Verification items for the finished model (mm, model axes). Face numbers are marked on the shaded views. A direction names the side the tool comes from. Round coordinates to 2 decimals unless told otherwise and drop trailing zeros. Write each loop counter-clockwise with the first axis right and the second up, starting at its lowest first coordinate (ties: lowest second). Pieces come first, ordered by that corner, then holes. Notation, with made-up numbers: M -31,82 L -5,82 A23 cw -5,95 Z; hole C 50.25,39.5 d1. An arc over 180 degrees is marked long. One line per question, with ' | ' between items.
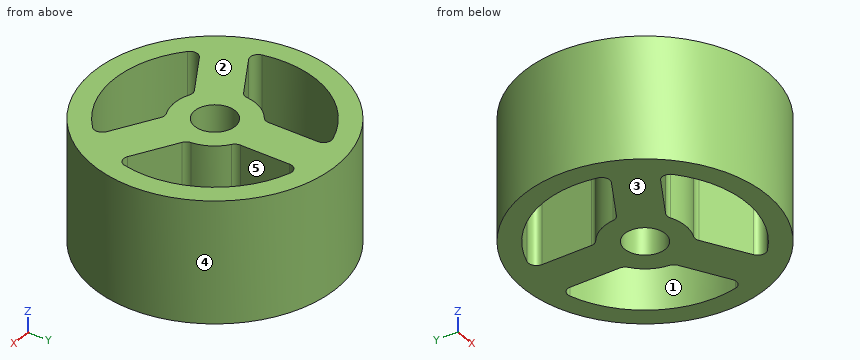
from build123d import *

# Parameters (mm, degrees)
SKETCH1_R           = 30
SKETCH1_R_2         = 25
SKETCH1_R_3         = 10
SKETCH1_R_4         = 5
BOSS_EXTRUDE1_DEPTH = 30


with BuildPart() as part:
    # Sketch1 → Boss-Extrude1 (new body)
    # profile 1 of 5: a face of its own
    with BuildSketch(Plane.XY):
        Circle(SKETCH1_R)
        Circle(SKETCH1_R_2, mode=Mode.SUBTRACT)
    # profile 2 of 5: a face of its own
    with BuildSketch(Plane.XY):
        with BuildLine():
            ThreePointArc((-7.608695652, 23.814024239), (-5.820464351, 23.524048006), (-5, 21.9089023))
            Line((-5, 21.9089023), (-5, 9.746794345))
            ThreePointArc((-5, 9.746794345), (-5.220486958, 8.833923416), (-5.833333333, 8.122328621))
            ThreePointArc((-5.833333333, 8.122328621), (0, 10), (5.833333333, 8.122328621))
            ThreePointArc((5.833333333, 8.122328621), (5.220486958, 8.833923416), (5, 9.746794345))
            Line((5, 9.746794345), (5, 21.9089023))
            ThreePointArc((5, 21.9089023), (5.820464351, 23.524048006), (7.608695652, 23.814024239))
            ThreePointArc((7.608695652, 23.814024239), (0, 25), (-7.608695652, 23.814024239))
        make_face()
    # profile 3 of 5: a face of its own
    with BuildSketch(Plane.XY):
        with BuildLine():
            ThreePointArc((-21.473665961, -6.624324131), (-23.282655349, -6.721354014), (-24.427897784, -5.317688395))
            ThreePointArc((-24.427897784, -5.317688395), (-21.650635095, -12.5), (-16.819202132, -18.496335844))
            ThreePointArc((-16.819202132, -18.496335844), (-17.462190998, -16.802693993), (-16.473665961, -15.284578169))
            Line((-16.473665961, -15.284578169), (-5.940971508, -9.203524191))
            ThreePointArc((-5.940971508, -9.203524191), (-5.040158614, -8.938036034), (-4.117476257, -9.112979166))
            ThreePointArc((-4.117476257, -9.112979166), (-8.660254038, -5), (-9.95080959, 0.990650545))
            ThreePointArc((-9.95080959, 0.990650545), (-10.260645572, 0.104112618), (-10.940971508, -0.543270153))
            Line((-10.940971508, -0.543270153), (-21.473665961, -6.624324131))
        make_face()
    # profile 4 of 5: a face of its own
    with BuildSketch(Plane.XY):
        with BuildLine():
            ThreePointArc((10.940971508, -0.543270153), (10.260645572, 0.104112618), (9.95080959, 0.990650545))
            ThreePointArc((9.95080959, 0.990650545), (9.987694827, 0.49593553), (10, 0))
            ThreePointArc((10, 0), (8.40162968, -5.423340181), (4.117476257, -9.112979166))
            ThreePointArc((4.117476257, -9.112979166), (5.040158614, -8.938036034), (5.940971508, -9.203524191))
            Line((5.940971508, -9.203524191), (16.473665961, -15.284578169))
            ThreePointArc((16.473665961, -15.284578169), (17.462190998, -16.802693993), (16.819202132, -18.496335844))
            ThreePointArc((16.819202132, -18.496335844), (21.650635095, -12.5), (24.427897784, -5.317688395))
            ThreePointArc((24.427897784, -5.317688395), (23.282655349, -6.721354014), (21.473665961, -6.624324131))
            Line((21.473665961, -6.624324131), (10.940971508, -0.543270153))
        make_face()
    # profile 5 of 5: a face of its own
    with BuildSketch(Plane.XY):
        Circle(SKETCH1_R_3)
        Circle(SKETCH1_R_4, mode=Mode.SUBTRACT)
    extrude(amount=BOSS_EXTRUDE1_DEPTH)


solid = part.part
1. Go/stop test with flat-tipped pins: P1, Ø10, axis at y = -17, z = 16.5, coming from the -X side; P2, Ø1, axis at y = -11, z = 25.5, coming from the -X side; P3, Ø1, axis at x = -17.5, y = -4, coming from the +Z side; P4, Ø6, axis at y = 16, z = 22, coming from the -X side. Record where each tip stops, or that it passes through.
Results:
P1: stops at x = -27.5 | P2: stops at x = -28.1 | P3: stops at z = 30 | P4: stops at x = -27.04
2. Tool access check on the marked faces 1 and 2. Record the directions out of +Z, -Z, +X, -X, +Y, -Y that give a thin tool (end or side, any length) a straight path to the whole face; none if there is none.
Results:
face 1: +Z, -Z | face 2: +Z, +X, -X, +Y, -Y
3. Thickness scan on line 1 (X direction, y = -6.5, z = 26.5); line 2 (X direction, y = 11, z = 13.25); line 3 (Y direction, x = 17, z = 9.75). Record the ranges inside material, lowest first.
Results:
line 1: x = -29.29 to -23.66, -21.26 to 21.26, 23.66 to 29.29 | line 2: x = -27.91 to -22.45, -5 to 5, 22.45 to 27.91 | line 3: y = -24.72 to -18.31, -15.72 to -4.04, 18.33 to 24.72
4. Section check D-D, the plane y = 17.5. Record the cut outline in (x, z).
Results:
outline: M -24.37,0 L -17.85,0 L -17.85,30 L -24.37,30 Z; M -5,0 L 5,0 L 5,30 L -5,30 Z; M 17.85,0 L 24.37,0 L 24.37,30 L 17.85,30 Z
5. Section check B-B, the plane y = -11.5. Record the cut outline in (x, z), then the cut area to 3 significant figures.
Results:
outline: M -27.71,0 L -9.92,0 L -9.92,30 L -27.71,30 Z; M 9.92,0 L 27.71,0 L 27.71,30 L 9.92,30 Z | area: 1,070 mm2
6. Mould release check, pull along Y, two halves, no side actions. Record for the marked faces 3, 4 and 5: pulls with the +Y half, pulls with the -Y half, needs draft (parallel to the pull), parting line crosses it, or undercut.
Results:
face 3: needs draft | face 4: parting line crosses it | face 5: undercut
7. Section check A-A, the plane x = 0. Record the cut outline in (y, z).
Results:
outline: M -30,0 L -25,0 L -25,30 L -30,30 Z; M -10,0 L -5,0 L -5,30 L -10,30 Z; M 5,0 L 30,0 L 30,30 L 5,30 Z
8. Section check C-C, the plane z = 19. Record the cut outline in (x, y).
Results:
outline: C 0,0 d60; hole M -24.43,-5.32 A2 ccw -21.47,-6.62 L -10.94,-0.54 A2 ccw -9.95,0.99 A10 cw -5.83,8.12 A2 ccw -5,9.75 L -5,21.91 A2 ccw -7.61,23.81 A25 ccw Z; hole M -16.82,-18.5 A25 ccw 16.82,-18.5 A2 ccw 16.47,-15.28 L 5.94,-9.2 A2 ccw 4.12,-9.11 A10 cw -4.12,-9.11 A2 ccw -5.94,-9.2 L -16.47,-15.28 A2 ccw Z; hole C 0,0 d10; hole M 5,9.75 A2 ccw 5.83,8.12 A10 cw 9.95,0.99 A2 ccw 10.94,-0.54 L 21.47,-6.62 A2 ccw 24.43,-5.32 A25 ccw 7.61,23.81 A2 ccw 5,21.91 Z
